from build123d import *

# Parameters (mm, degrees)
F0_W     = 203.2
F0_H     = 254
F1_DEPTH = 6.35
F2_W     = 203.2
F2_H     = 6.35
F3_DEPTH = 44.45
F4_R     = 3.175
F6_DEPTH = 25.4
F7_DEPTH = 25.4
F8_R     = 1.27


with BuildPart() as f1:
    # F0 (on Top) → F1 (new body)
    with BuildSketch(Plane.XY):
        Rectangle(F0_W, F0_H)
    extrude(amount=F1_DEPTH)

    # F2 (on face) → F3 (join)
    with BuildSketch(Plane.XY.offset(6.35)):
        with Locations((0, 123.825)):
            Rectangle(F2_W, F2_H)
    extrude(amount=F3_DEPTH)

    # F4
    f4_edges = [f1.edges().sort_by_distance(p)[0] for p in [
        (0, 120.65, 6.35),
        (0, 127, 0),
    ]]
    fillet(f4_edges, radius=F4_R)

    # F5 (on face) → F6 (cut)
    with BuildSketch(Plane.XY.offset(6.35)):
        with BuildLine():
            ThreePointArc((-69.85, -43.65625), (-64.798606, -45.748606), (-62.70625, -50.8))
            ThreePointArc((-62.70625, -50.8), (-64.798606, -55.851394), (-69.85, -57.94375))
            Line((-69.85, -57.94375), (-44.45, -57.94375))
            ThreePointArc((-44.45, -57.94375), (-51.59375, -50.8), (-44.45, -43.65625))
            Line((-44.45, -43.65625), (-69.85, -43.65625))
        make_face()
        with BuildLine():
            ThreePointArc((-37.30625, -50.8), (-39.398606, -45.748606), (-44.45, -43.65625))
            ThreePointArc((-44.45, -43.65625), (-51.59375, -50.8), (-44.45, -57.94375))
            ThreePointArc((-44.45, -57.94375), (-39.398606, -55.851394), (-37.30625, -50.8))
        make_face()
        with BuildLine():
            ThreePointArc((-69.85, -57.94375), (-64.798606, -55.851394), (-62.70625, -50.8))
            ThreePointArc((-62.70625, -50.8), (-64.798606, -45.748606), (-69.85, -43.65625))
            ThreePointArc((-69.85, -43.65625), (-76.99375, -50.8), (-69.85, -57.94375))
        make_face()
    extrude(amount=-F6_DEPTH, mode=Mode.SUBTRACT)

    # F5 (on face) → F7 (cut)
    with BuildSketch(Plane.XY.offset(6.35)):
        with BuildLine():
            ThreePointArc((-69.85, -57.94375), (-64.798606, -55.851394), (-62.70625, -50.8))
            ThreePointArc((-62.70625, -50.8), (-64.798606, -45.748606), (-69.85, -43.65625))
            ThreePointArc((-69.85, -43.65625), (-76.99375, -50.8), (-69.85, -57.94375))
        make_face()
        with BuildLine():
            ThreePointArc((-69.85, -43.65625), (-64.798606, -45.748606), (-62.70625, -50.8))
            ThreePointArc((-62.70625, -50.8), (-64.798606, -55.851394), (-69.85, -57.94375))
            Line((-69.85, -57.94375), (-44.45, -57.94375))
            ThreePointArc((-44.45, -57.94375), (-51.59375, -50.8), (-44.45, -43.65625))
            Line((-44.45, -43.65625), (-69.85, -43.65625))
        make_face()
        with BuildLine():
            ThreePointArc((-37.30625, -50.8), (-39.398606, -45.748606), (-44.45, -43.65625))
            ThreePointArc((-44.45, -43.65625), (-51.59375, -50.8), (-44.45, -57.94375))
            ThreePointArc((-44.45, -57.94375), (-39.398606, -55.851394), (-37.30625, -50.8))
        make_face()
        with BuildLine():
            ThreePointArc((-69.85, 43.65625), (-64.798606, 45.748606), (-62.70625, 50.8))
            ThreePointArc((-62.70625, 50.8), (-64.798606, 55.851394), (-69.85, 57.94375))
            ThreePointArc((-69.85, 57.94375), (-76.99375, 50.8), (-69.85, 43.65625))
        make_face()
        with BuildLine():
            ThreePointArc((-69.85, 57.94375), (-64.798606, 55.851394), (-62.70625, 50.8))
            ThreePointArc((-62.70625, 50.8), (-64.798606, 45.748606), (-69.85, 43.65625))
            Line((-69.85, 43.65625), (-44.45, 43.65625))
            ThreePointArc((-44.45, 43.65625), (-51.59375, 50.8), (-44.45, 57.94375))
            Line((-44.45, 57.94375), (-69.85, 57.94375))
        make_face()
        with BuildLine():
            ThreePointArc((-37.30625, 50.8), (-39.398606, 55.851394), (-44.45, 57.94375))
            ThreePointArc((-44.45, 57.94375), (-51.59375, 50.8), (-44.45, 43.65625))
            ThreePointArc((-44.45, 43.65625), (-39.398606, 45.748606), (-37.30625, 50.8))
        make_face()
    extrude(amount=-F7_DEPTH, mode=Mode.SUBTRACT)

    # F8
    f8_edges = [f1.edges().sort_by_distance(p)[0] for p in [
        (0, -127, 6.35),
        (0, -127, 0),
        (0, 120.65, 50.8),
        (0, 127, 50.8),
    ]]
    fillet(f8_edges, radius=F8_R)


solid = f1.part
CAD build for the part. Positions are in the model's coordinates, mm. A direction names the side the tool comes from. Coordinates: 2 decimals unless noted, no trailing zeros. Write each loop counter-clockwise with the first axis right and the second up, starting at its lowest first coordinate (ties: lowest second). Pieces come first, ordered by that corner, then holes. Notation, with made-up numbers: M 33,63.5 L 66,63.5 A12 ccw 66,85.5 Z; hole C 27.25,7 d7. An arc over 180 degrees is marked long. Return JSON: item names as keys, results as strings.
Item 1: Drop a flat-ended pin along its axis: pin 1 Ø8 at (x, y) = (26, 78) entering from +Z. Give the stop position or say it passes through.
Findings below:
{"pin 1": "stops at z = 6.35"}
Item 2: Two-plate mould, pull along Y, no slides. Class faces 4 (the flat face through (-1, 127, 26)), 5 (the cylindrical face through (-76.99, -50.64, 3.22)), 6 (the flat face through (101.6, 28, 3)), 7 (the flat face through (-1, 120.65, 29)): +Y half, -Y half, draft (parallel to the pull), parting line (faces both ways), or undercut.
Findings below:
{"face 4": "+Y half", "face 5": "undercut", "face 6": "draft", "face 7": "-Y half"}
Item 3: Slice it at C-C, the plane x = -41.5. Write the cut outline in (y, z) (3 decimals), and give its area (3 significant figures).
Findings below:
{"outline": "M -127,1.27 A1.27 ccw -125.73,0 L -57.306,0 L -57.306,6.35 L -125.73,6.35 A1.27 ccw -127,5.08 Z; M -44.294,0 L 44.294,0 L 44.294,6.35 L -44.294,6.35 Z; M 57.306,0 L 123.825,0 A3.175 ccw 127,3.175 L 127,49.53 A1.27 ccw 125.73,50.8 L 121.92,50.8 A1.27 ccw 120.65,49.53 L 120.65,9.525 A3.175 cw 117.475,6.35 L 57.306,6.35 Z", "area": "1,730 mm2"}
Item 4: Slice it at B-B, the plane x = -84. Write the cut outline in (y, z) (3 decimals), and give its area (3 significant figures).
Findings below:
{"outline": "M -127,1.27 A1.27 ccw -125.73,0 L 123.825,0 A3.175 ccw 127,3.175 L 127,49.53 A1.27 ccw 125.73,50.8 L 121.92,50.8 A1.27 ccw 120.65,49.53 L 120.65,9.525 A3.175 cw 117.475,6.35 L -125.73,6.35 A1.27 ccw -127,5.08 Z", "area": "1,890 mm2"}
Item 5: Which spindle directions (+Z, -Z, +X, -X, +Y, -Y) get a long thin tool onto all of the face, cutting with end or side? Do faces 1 (the flat face through (-1, -2, 6.35)), 2 (the flat face through (-1, 1, 0)), 3 (the flat face through (-57, -57.944, 3)). Say none if no direction does.
Findings below:
{"face 1": "+Z, +X, -X, -Y", "face 2": "-Z, +X, -X, +Y, -Y", "face 3": "+Z, -Z"}
Item 6: Slice it at A-A, the plane y = 47.5. Write the cut outline in (x, z), and give its area (3 significant figures).
Findings below:
{"outline": "M -101.6,0 L -76.19,0 L -76.19,6.35 L -101.6,6.35 Z; M -38.11,0 L 101.6,0 L 101.6,6.35 L -38.11,6.35 Z", "area": "1,050 mm2"}
Item 7: Slice it at D-D, the plane z = 19. Write the cut outline in (x, y).
Findings below:
{"outline": "M -101.6,120.65 L 101.6,120.65 L 101.6,127 L -101.6,127 Z"}
Item 8: Probe line 1 (Y direction, x = 69, z = 36); line 2 (Z direction, x = -47, y = -86.5). List the from-to ranges inside material, lowest first. Write a range as from..to.
Findings below:
{"line 1": "y = 120.65..127", "line 2": "z = 0..6.35"}
